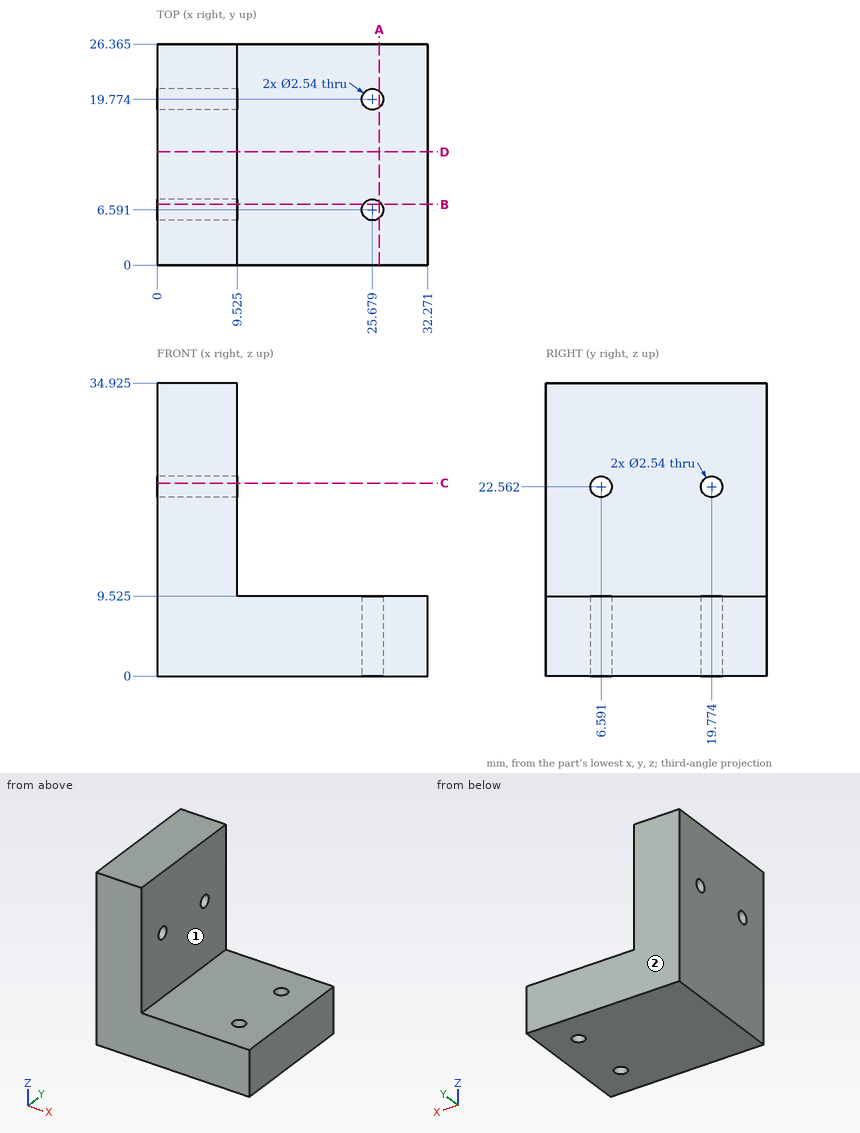
Part print with two shaded views. Sizes in mm from the minimum x, y, z corner. A direction names the side the tool comes from. Round coordinates to 2 decimals unless told otherwise and drop trailing zeros. Order: outer loops, then holes, each group sorted by start corner. A loop starts at its lowest first (then second) coordinate and runs counter-clockwise, first axis right, second up.
(1) Band-saw the part on B-B (y = 7.25). List the corners of the cut face in (x, z) (1 decimal), then the cut area to 3 significant figures.
(2) 3-axis set-ups, long thin cutter, end or side, ignore diameter. For the marked faces 1 and 2: which of +Z, -Z, +X, -X, +Y, -Y reach the whole face in a straight line?
(3) Band-saw the part on C-C (z = 23). List the corners of the cut face in (x, y) (1 decimal), then the cut area to 3 significant figures.
(4) Band-saw the part on D-D (y = 13.5). List the corners of the cut face in (x, z) (1 decimal), then the cut area to 3 significant figures.
(5) Pin check, flat tips, straight feed: pin 1 (6 mm diameter, centred on y = 19.5, z = 12, fed in from -X); pin 2 (6 mm diameter, centred on x = 19.5, y = 18, fed in from +Z) (3 decimals); pin 3 (1.5 mm diameter, centred on y = 6.59, z = 22.56, fed in from -X); pin 4 (3.5 mm diameter, centred on y = 19.77, z = 22.56, fed in from +X) (3 decimals). Stop position of each tip, or through.
(6) Drill centre line: line 1 (X direction, y = 10, z = 28) (1 decimal). Where is it in solid material? Low to high.
(7) Band-saw the part on A-A (x = 26.5). List the corners of the cut face in (y, z) (1 decimal).
Verdict:
1. outline: (0, 0) - (24.6, 0) - (24.6, 9.5) - (9.5, 9.5) - (9.5, 21.5) - (0, 21.5) - close; (0, 23.6) - (9.5, 23.6) - (9.5, 34.9) - (0, 34.9) - close; (26.8, 0) - (32.3, 0) - (32.3, 9.5) - (26.8, 9.5) - close
1. area: 508 mm2
2. face 1: +Z, +X, +Y, -Y
2. face 2: +Z, -Z, +X, -X, +Y
3. outline: (0, 0) - (9.5, 0) - (9.5, 5.4) - (0, 5.4) - close; (0, 7.8) - (9.5, 7.8) - (9.5, 18.6) - (0, 18.6) - close; (0, 21) - (9.5, 21) - (9.5, 26.4) - (0, 26.4) - close
3. area: 206 mm2
4. outline: (0, 0) - (32.3, 0) - (32.3, 9.5) - (9.5, 9.5) - (9.5, 34.9) - (0, 34.9) - close
4. area: 549 mm2
5. pin 1: stops at x = 0
5. pin 2: stops at z = 9.525
5. pin 3: passes through
5. pin 4: stops at x = 9.525
6. line 1: x = 0 to 9.5
7. outline: (0, 0) - (5.6, 0) - (5.6, 9.5) - (0, 9.5) - close; (7.6, 0) - (18.8, 0) - (18.8, 9.5) - (7.6, 9.5) - close; (20.7, 0) - (26.4, 0) - (26.4, 9.5) - (20.7, 9.5) - close
